from build123d import *

# Parameters (mm, degrees)
F0_W     = 57.15
F0_H     = 68.072
F1_DEPTH = 14.224
F2_W     = 34.925
F2_H     = 31.75
F3_DEPTH = 26.924
F5_DEPTH = 1.5875
F7_D     = 3.7973
F7_DEPTH = 14.605
F7_TIP   = 1.1408240143


with BuildPart() as f1:
    # F0 (on Front) → F1 (new body, symmetric)
    with BuildSketch(Plane.XZ):
        Rectangle(F0_W, F0_H)
    extrude(amount=F1_DEPTH, both=True)

    # F2 (on Front) → F3 (join, symmetric)
    with BuildSketch(Plane.XZ):
        Rectangle(F2_W, F2_H)
    extrude(amount=F3_DEPTH, both=True)

    # F4 (on face) → F5 (join)
    with BuildSketch(Plane(origin=(0, 0, -34.036), x_dir=(1, 0, 0), z_dir=(0, 0, -1))):
        with BuildLine():
            Line((-28.575, -14.224), (-28.575, 14.224))
            ThreePointArc((-28.575, 14.224), (-39.624, 0), (-28.575, -14.224))
        make_face()
        with BuildLine():
            ThreePointArc((28.575, -14.224), (39.624, 0), (28.575, 14.224))
            Line((28.575, 14.224), (28.575, -14.224))
        make_face()
    extrude(amount=-F5_DEPTH)

    # F7
    with Locations(Plane(origin=(0, 0, -34.036), x_dir=(1, 0, 0), z_dir=(0, 0, -1))):
        with Locations((-35.687, 0), (35.687, 0)):
            Hole(F7_D / 2, depth=F7_DEPTH)
            with Locations((0, 0, -(F7_DEPTH + F7_TIP / 2))):  # 118° drill point
                Cone(0, F7_D / 2, F7_TIP, mode=Mode.SUBTRACT)


solid = f1.part
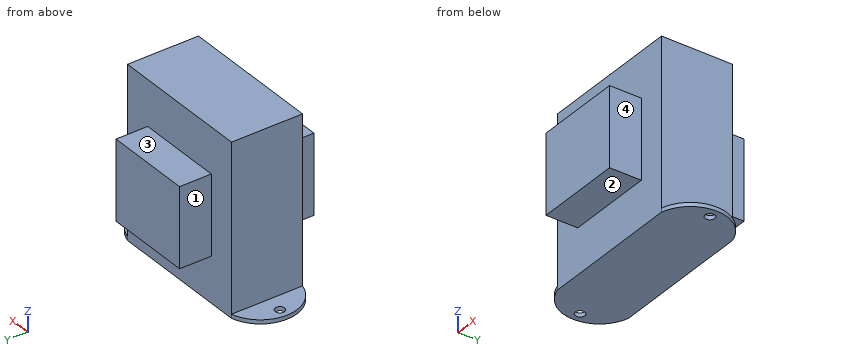
Verification items for the finished model (mm, model axes). Face numbers are marked on the shaded views. A direction names the side the tool comes from. Coordinates: 2 decimals unless noted, no trailing zeros. Order: outer loops, then holes, each group sorted by start corner. A loop starts at its lowest first (then second) coordinate and runs counter-clockwise, first axis right, second up. Notation, with made-up numbers: M 9.5,76 L 25.5,76 A22 cw 25.5,85 Z; hole C 62,-38.5 d4. An arc over 180 degrees is marked long. One line per item, written item: value. Start each with the question number.
Item 1: Depth check by flat-ended pin: P1, Ø4, axis at y = -23.5, z = -5.5, coming from the +X side; P2, Ø4, axis at x = 2, y = -20, coming from the -Z side (3 decimals); P3, Ø6.5, axis at x = -7.5, y = 23, coming from the +Z side (3 decimals); P4, Ø4.5, axis at x = 35.687, y = 0, coming from the -Z side. Enter the tip coordinate at first touch or a pass-through.
Item 2: Sectioned sample at A-A on z = 13. Record the cut outline in (x, y) (1 decimal), then the cut area to 3 significant figures.
Item 3: Thickness scan on probe 1 along Z at (x, y) = (17, 16) (3 decimals); probe 2 along X at (y, z) = (8.5, -20) (3 decimals); probe 3 along Y at (x, z) = (7, 29.5). Record the ranges inside material, lowest first.
Item 4: Sectioned sample at B-B on y = 11. Record the cut outline in (x, z) (1 decimal), then the cut area to 3 significant figures.
Item 5: Sectioned sample at C-C on x = -25. Record the cut outline in (y, z).
Item 6: Access from +Z, -Z, +X, -X, +Y, -Y to the whole of each face (thin tool, end or side, straight path). Record for the marked faces 1, 2, 3 and 4.
Item 7: Sectioned sample at D-D on y = -3. Record the cut outline in (x, z) (1 decimal).
Calculated:
1. P1: x = 17.46
1. P2: z = -15.875
1. P3: z = 15.875
1. P4: z = -34.04
2. outline: M -28.6,-14.2 L -17.5,-14.2 L -17.5,-26.9 L 17.5,-26.9 L 17.5,-14.2 L 28.6,-14.2 L 28.6,14.2 L 17.5,14.2 L 17.5,26.9 L -17.5,26.9 L -17.5,14.2 L -28.6,14.2 Z
2. area: 2,510 mm^2
3. probe 1: -15.875 to 15.875
3. probe 2: -28.575 to 28.575
3. probe 3: -14.22 to 14.22
4. outline: M -34.7,-34 L 34.7,-34 L 34.7,-32.4 L 28.6,-32.4 L 28.6,34 L -28.6,34 L -28.6,-32.4 L -34.7,-32.4 Z
4. area: 3,910 mm^2
5. outline: M -14.22,-34.04 L 14.22,-34.04 L 14.22,34.04 L -14.22,34.04 Z
6. face 1: +Z, -Z, -X, +Y
6. face 2: -Z, +X, -X, -Y
6. face 3: +Z, +X, -X, +Y
6. face 4: +Z, -Z, +X, -Y
7. outline: M -39.3,-34 L 39.3,-34 L 39.3,-32.4 L 28.6,-32.4 L 28.6,34 L -28.6,34 L -28.6,-32.4 L -39.3,-32.4 Z
